```python
from build123d import *

# Parameters (mm, degrees)
SKETCH1_W           = 24
SKETCH1_H           = 17.7
BOSS_EXTRUDE1_DEPTH = 3
SKETCH2_R           = 2.1
BOSS_EXTRUDE2_DEPTH = 3
BOSS_EXTRUDE3_DEPTH = 3
CHAMFER1_SIZE       = 6
CHAMFER1_SIZE2      = 3
CHAMFER2_SIZE       = 3
CHAMFER2_SIZE2      = 6
FILLET1_R           = 2


with BuildPart() as part:
    # Sketch1 → Boss-Extrude1 (new body)
    with BuildSketch(Plane(origin=(0, 0, 0), x_dir=(1, 0, 0), z_dir=(0, 1, 0))):
        with Locations((0, -8.85)):
            Rectangle(SKETCH1_W, SKETCH1_H)
        with BuildLine():
            Line((-9.34985398, -6.208693331), (-8, -7.341355308))
            Line((-8, -7.341355308), (-6.65014602, -6.208693331))
            ThreePointArc((-6.65014602, -6.208693331), (-8, -2.5), (-9.34985398, -6.208693331))
        make_face(mode=Mode.SUBTRACT)
        with BuildLine():
            Line((6.65014602, -6.208693331), (8, -7.341355308))
            Line((8, -7.341355308), (9.34985398, -6.208693331))
            ThreePointArc((9.34985398, -6.208693331), (8, -2.5), (6.65014602, -6.208693331))
        make_face(mode=Mode.SUBTRACT)
        with BuildLine():
            Line((-1.34985398, -14.208693331), (0, -15.341355308))
            Line((0, -15.341355308), (1.34985398, -14.208693331))
            ThreePointArc((1.34985398, -14.208693331), (0, -10.5), (-1.34985398, -14.208693331))
        make_face(mode=Mode.SUBTRACT)
    extrude(amount=BOSS_EXTRUDE1_DEPTH)

    # Sketch2 → Boss-Extrude2 (add)
    with BuildSketch(Plane.XY):
        Polygon((12, 0), (-12, 0), (-12, 37.9), (-24.1, 37.9), (-24.1, 46.1), (-12, 46.1), (4, 46.1), (4, 31.1), (12, 31.1), align=None)
        with Locations((-20, 42)):
            Circle(SKETCH2_R, mode=Mode.SUBTRACT)
        with Locations((-4, 42)):
            Circle(SKETCH2_R, mode=Mode.SUBTRACT)
    extrude(amount=-BOSS_EXTRUDE2_DEPTH)

    # Sketch3 → Boss-Extrude3 (add, symmetric)
    with BuildSketch(Plane(origin=(0, 0, 0), x_dir=(0, 0, -1), z_dir=(1, 0, 0))):
        Polygon((0, 3), (-8, 3), (0, 38), align=None)
    extrude(amount=BOSS_EXTRUDE3_DEPTH, both=True)

    # Chamfer1
    chamfer1_edges = [part.edges().sort_by_distance(p)[0] for p in [
        (12, 1.5, 17.7),
    ]]
    chamfer1_side = [part.faces().sort_by_distance(p)[0] for p in [
        (0, 1.5, 17.7),
    ]]
    chamfer(chamfer1_edges, length=CHAMFER1_SIZE, length2=CHAMFER1_SIZE2, reference=chamfer1_side[0])

    # Chamfer2
    chamfer2_edges = [part.edges().sort_by_distance(p)[0] for p in [
        (-12, 1.5, 17.7),
    ]]
    chamfer2_side = [part.faces().sort_by_distance(p)[0] for p in [
        (-12, 1.5, 17.26815512),
    ]]
    chamfer(chamfer2_edges, length=CHAMFER2_SIZE, length2=CHAMFER2_SIZE2, reference=chamfer2_side[0])

    # Fillet1
    fillet1_edges = [part.edges().sort_by_distance(p)[0] for p in [
        (12, 31.1, -1.5),
        (-12, 37.9, -1.5),
        (-24.1, 37.9, -1.5),
        (-24.1, 46.1, -1.5),
        (4, 46.1, -1.5),
        (4, 31.1, -1.5),
    ]]
    fillet(fillet1_edges, radius=FILLET1_R)


solid = part.part
```
Geometry check sheet. Reference: the model listing, model coordinates, mm. A direction names the side the tool comes from. Round coordinates to 2 decimals unless told otherwise and drop trailing zeros. Order: outer loops, then holes, each group sorted by start corner. A loop starts at its lowest first (then second) coordinate and runs counter-clockwise, first axis right, second up. Notation, with made-up numbers: (51.25, 20.5) - (59.25, 20.5) arc R22 ccw to (59.25, 52.5) - close; hole circle Ø1 at (81, 10). An arc over 180 degrees is marked (long way). Use a Markdown table: item, result. Add a question column.
(1) Tool access check on faces 1 (the flat face through (0, 3, 9)), 2 (the cylindrical face through (-12.57, 37.3, -1.52)), 3 (the flat face through (7.32, 1.48, 6.77)), 4 (the flat face through (-3, 13, 2)), 5 (the flat face through (8, 31.1, -1)). Record the directions out of +Z, -Z, +X, -X, +Y, -Y that give a thin tool (end or side, any length) a straight path to the whole face; none if there is none.
(2) Sectioned sample at D-D, the plane z = 4.6. Enter the section's corners in (x, y) (3 decimals).
(3) Release check for a two-part mould opening along Z. For faces 6 (the cylindrical face through (-19.031, 40.137, -1.479)), 7 (the flat face through (-7.33, 1.48, 6.78)), 8 (the flat face through (0.67, 1.48, 14.78)), 9 (the flat face through (0, 1, 17.7)) record: pulls with the +Z half, pulls with the -Z half, needs draft (parallel to the pull), parting line crosses it, or undercut.
(4) Sectioned sample at C-C, the plane y = 42. Enter the section's corners in (x, z).
(5) Material ranges on line 1 along X through (y, z) = (1.1, 4.6); line 2 along X through (y, z) = (1.6, 12.6); line 3 along Z through (x, y) = (-3.5, 30.5), recorded low to high. Write a range as [from, to].
(6) Sectioned sample at B-B, the plane x = -4. Enter the section's corners in (y, z).
(7) Sectioned sample at A-A, the plane z = 12.6. Enter the section's corners in (x, y).
(8) Depth check by flat-ended pin: pin 1 (1.5 mm diameter, centred on x = 7.5, z = -1.5, fed in from +Y); pin 2 (1.5 mm diameter, centred on y = 40.5, z = -2, fed in from +X); pin 3 (9 mm diameter, centred on y = 13.5, z = 3.5, fed in from -X). Enter the tip coordinate at first touch or a pass-through.
Answers below:
| question | item | result |
|---|---|---|
| 1 | face 1 | +Z, +Y |
| 1 | face 2 | +Z, -Z, -X, -Y |
| 1 | face 3 | +Y, -Y |
| 1 | face 4 | +Z, -X, +Y |
| 1 | face 5 | +Z, -Z, +X, +Y |
| 2 | outline | (-12, 0) - (-10.1, 0) - (-10.1, 3) - (-12, 3) - close; (-5.9, 0) - (5.9, 0) - (5.9, 3) - (3, 3) - (3, 17.875) - (-3, 17.875) - (-3, 3) - (-5.9, 3) - close; (10.1, 0) - (12, 0) - (12, 3) - (10.1, 3) - close |
| 3 | face 6 | needs draft |
| 3 | face 7 | undercut |
| 3 | face 8 | undercut |
| 3 | face 9 | pulls with the +Z half |
| 4 | outline | (-24.1, -3) - (-22.1, -3) - (-22.1, 0) - (-24.1, 0) - close; (-17.9, -3) - (-6.1, -3) - (-6.1, 0) - (-17.9, 0) - close; (-1.9, -3) - (4, -3) - (4, 0) - (-1.9, 0) - close |
| 5 | line 1 | [-12, -10.1], [-5.9, 5.9], [10.1, 12] |
| 5 | line 2 | [-12, -2.1], [2.1, 12] |
| 5 | line 3 | [-3, 0] |
| 6 | outline | (0, -3) - (39.9, -3) - (39.9, 0) - (3, 0) - (3, 17.7) - (0, 17.7) - close; (44.1, -3) - (46.1, -3) - (46.1, 0) - (44.1, 0) - close |
| 7 | outline | (-12, 0) - (-2.1, 0) - (-2.1, 3) - (-12, 3) - close; (2.1, 0) - (12, 0) - (12, 3) - (2.1, 3) - close |
| 8 | pin 1 | y = 31.1 |
| 8 | pin 2 | x = 4 |
| 8 | pin 3 | x = -12 |
